from build123d import *


with BuildPart() as part:
    # Sketch1 → Revolve1 (revolve)
    with BuildSketch(Plane(origin=(0, 0, 0), x_dir=(0, 0, -1), z_dir=(1, 0, 0)), mode=Mode.PRIVATE) as revolve1_sk:
        with BuildLine():
            Line((0, 24.60625), (4.8815625, 24.60625))
            ThreePointArc((4.8815625, 24.60625), (6.948032483, 23.264493972), (6.563159633, 20.83087931))
            Line((6.563159633, 20.83087931), (3.175, 17.065625))
            Line((3.175, 17.065625), (3.175, 14.2875))
            ThreePointArc((3.175, 14.2875), (5.060465212, 11.001230365), (5.715, 7.269457141))
            Line((5.715, 7.269457141), (5.715, 4.826))
            Line((5.715, 4.826), (10.31875, 4.826))
            Line((10.31875, 4.826), (10.31875, 3.175))
            Line((10.31875, 3.175), (0, 3.175))
            Line((0, 3.175), (0, 24.60625))
        make_face()
    revolve(revolve1_sk.sketch.rotate(Axis((0, 0, -10.31875), (0, 0, 1)), 90), axis=Axis((0, 0, -10.31875), (0, 0, 1)))

    # Mirror1: part across plane


with BuildPart() as part_1:
    add(part.part)
    add(part.part.mirror(Plane.XY))


solid = part_1.part
Work out the finished part from the listing and answer in its coordinate system (mm). A direction names the side the tool comes from. Give positions to 0.01 mm unless a question says otherwise; leave off trailing zeros. Use a Markdown table: item, result. Add a question column.
1) Which of the six approach directions +Z, -Z, +X, -X, +Y, -Y give full straight-line access (tool end or side, diameter ignored) to faces 1 (the flat face through (4, 14, 3.175)), 2 (the flat face through (4, 14, -3.175)), 3 (the flat face through (1.14, 3.15, -10.319))?
2) Each of these flat-tipped pins is pushed along its axis until it touches: P1, Ø12, axis at x = 2, y = 12, coming from the +Z side (3 decimals); P2, Ø6, axis at x = 6.5, z = -6, coming from the +Y side; P3, Ø5, axis at x = -17.5, z = -7, coming from the -Y side. Where does it stop, or does it pass through?
3) Consider line 1 along Y through (x, z) = (0, 7.5) (3 decimals); line 2 along Y through (x, z) = (0, -4) (3 decimals); line 3 along Y through (x, z) = (0, -3.5) (3 decimals). Determine where each line is inside the solid, lowest interval first.
4) For a pull along X with two mould halves and no side action, classify faces 4 (the flat face through (1.14, 3.15, 10.319)), 5 (the conical face through (3.7, 16.8, 3.3)) as +X half, -X half, draft (parallel to the pull), parting line (faces both ways), or undercut.
Reported:
| question | item | result |
|---|---|---|
| 1 | face 1 | +Z |
| 1 | face 2 | -Z |
| 1 | face 3 | -Z, +X, -X, +Y, -Y |
| 2 | P1 | stops at z = 5.715 |
| 2 | P2 | stops at y = 24.33 |
| 2 | P3 | stops at y = -19.02 |
| 3 | line 1 | y = -4.826 to -3.175, 3.175 to 4.826 |
| 3 | line 2 | y = -24.606 to -17.982, -13.158 to -3.175, 3.175 to 13.158, 17.982 to 24.606 |
| 3 | line 3 | y = -24.606 to -17.427, -13.878 to -3.175, 3.175 to 13.878, 17.427 to 24.606 |
| 4 | face 4 | draft |
| 4 | face 5 | undercut |
